Verification items for this drawing (mm, ordinates from the low corner). Give positions to 0.01 mm unless a question says otherwise; leave off trailing zeros. Loops run counter-clockwise (first coordinate to the right, second up) from the corner with the lowest first, then second, coordinate; pieces in that order, holes last. Notation, with made-up numbers: (-21.5, -4) -> (-9.5, -4) arc R9 cw to (-9.5, 6) -> close; hole circle Ø7 at (15, -11.5). An arc over 180 degrees is marked (long way). Answer as a JSON object with one key per item and string values.
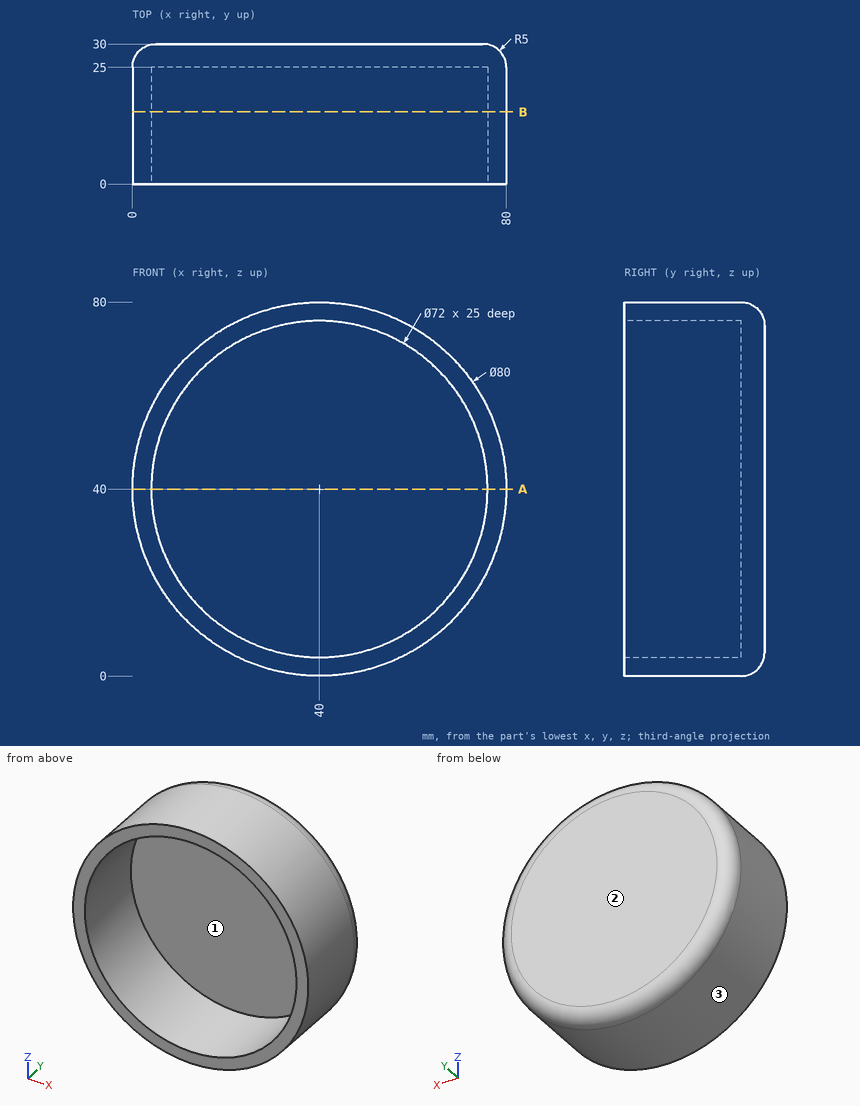
1) Depth check by flat-ended pin: P1, Ø3, axis at x = 37, y = 12.5, coming from the -Z side; P2, Ø8, axis at x = 50.5, y = 6, coming from the +Z side; P3, Ø4, axis at y = 16.5, z = 16, coming from the -X side. Enter the tip coordinate at first touch or a pass-through.
Geometry check:
{"P1": "stops at z = 0.03", "P2": "stops at z = 79.47", "P3": "stops at x = 6.59"}
2) Draft check along Z on the marked faces 1, 2 and 3. Enter one of: pulls with the +Z half, pulls with the -Z half, needs draft (parallel to the pull), parting line crosses it, or undercut.
Geometry check:
{"face 1": "undercut", "face 2": "needs draft", "face 3": "parting line crosses it"}
3) Material ranges on line 1 along X through (y, z) = (18.5, 40); line 2 along Y through (x, z) = (38, 64); line 3 along X through (y, z) = (3.5, 32.5), recorded low to high. Write a range as from..to.
Geometry check:
{"line 1": "x = 0..4, 76..80", "line 2": "y = 25..30", "line 3": "x = 0.71..4.79, 75.21..79.29"}
4) Section check B-B on y = 15.5. Record the cut outline in (x, z), plus the area to 3 significant figures.
Geometry check:
{"outline": "circle Ø80 at (40, 40); hole circle Ø72 at (40, 40)", "area": "955 mm2"}
5) Section check A-A on z = 40. Record the cut outline in (x, y), plus the area to 3 significant figures.
Geometry check:
{"outline": "(0, 0) -> (4, 0) -> (4, 25) -> (76, 25) -> (76, 0) -> (80, 0) -> (80, 25) arc R5 ccw to (75, 30) -> (5, 30) arc R5 ccw to (0, 25) -> close", "area": "589 mm2"}
